Job drawing, mm, ordinate dimensions from the low corner. One solid piece. A direction names the side the tool comes from. Give positions to 0.01 mm unless a question says otherwise; leave off trailing zeros. Write each loop counter-clockwise with the first axis right and the second up, starting at its lowest first coordinate (ties: lowest second). Pieces come first, ordered by that corner, then holes. Notation, with made-up numbers: (37, 44.5) - (53, 44.5) arc R19 ccw to (53, 50.5) - close; hole circle Ø4 at (-16, 35). An arc over 180 degrees is marked (long way). Put each result on its own line as item: value. Start each with the question number.
1. Wall check: line 1 (Y direction, x = 131, z = 4.5); line 2 (X direction, y = 82, z = 46); line 3 (Z direction, x = 114, y = 110). Give the ranges that are in metal, low to high.
2. Cut at A-A on x = 74.5. List the corners of the cut face in (y, z).
3. Tool access for the marked faces 4 and 5: list every direction of +Z, -Z, +X, -X, +Y, -Y with a clear straight run to the whole face (end or side of a thin tool).
4. Cut at B-B on y = 38. List the corners of the cut face in (x, z), and give its area (3 significant figures).
5. Cut at C-C on z = 54. List the corners of the cut face in (x, y), and give its area (3 significant figures).
6. Cut at D-D on z = 74.5. List the corners of the cut face in (x, y), and give its area (3 significant figures).
7. Drop flat-ended pins along their axis: pin 1 (3 mm diameter, centred on x = 83.5, z = 85.5, fed in from -Y); pin 2 (6 mm diameter, centred on x = 105, y = 30, fed in from +Z). Give the stop position or say it passes through.
8. Mould opens along Y. For the marked faces 1, 2 and 3 say: +Y half, -Y half, draft (parallel to the pull), parting line (faces both ways), or undercut.
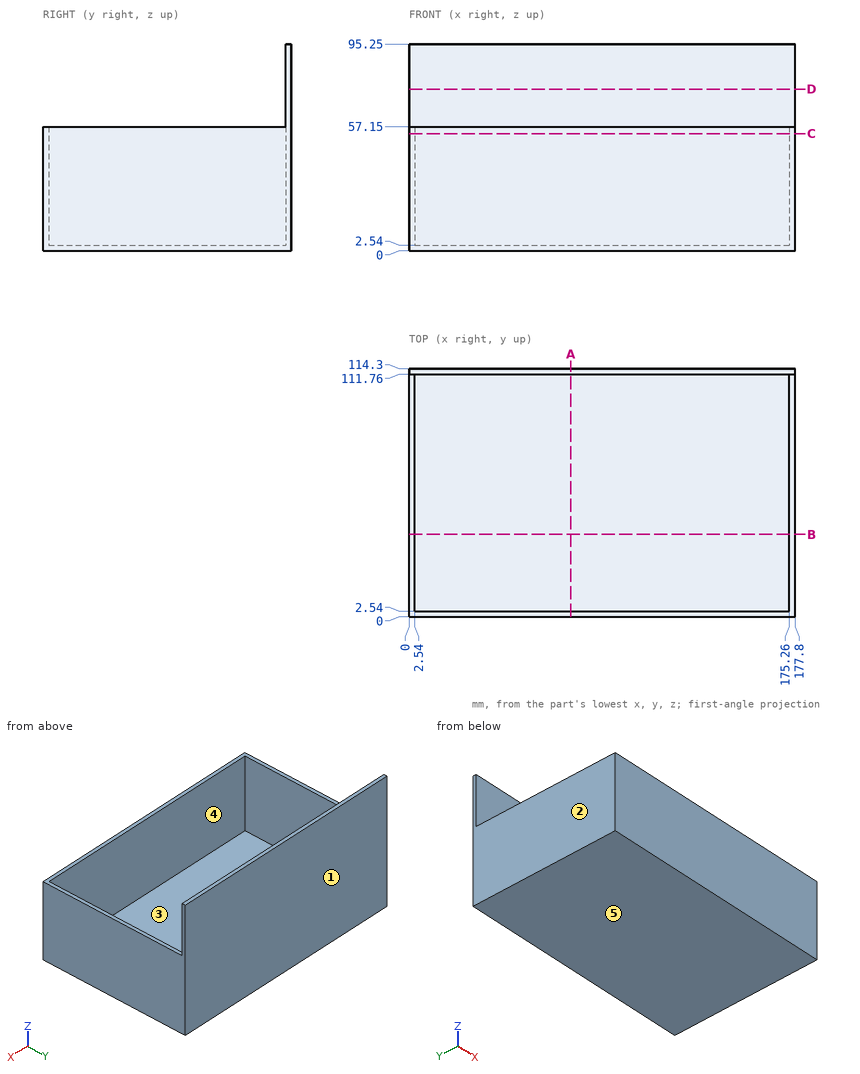
Report:
1. line 1: y = 0 to 2.54, 111.76 to 114.3
1. line 2: x = 0 to 2.54, 175.26 to 177.8
1. line 3: z = 0 to 2.54
2. outline: (0, 0) - (114.3, 0) - (114.3, 95.25) - (111.76, 95.25) - (111.76, 2.54) - (2.54, 2.54) - (2.54, 57.15) - (0, 57.15) - close
3. face 4: +Z
3. face 5: -Z, +X, -X, +Y, -Y
4. outline: (0, 0) - (177.8, 0) - (177.8, 57.15) - (175.26, 57.15) - (175.26, 2.54) - (2.54, 2.54) - (2.54, 57.15) - (0, 57.15) - close
4. area: 729 mm²
5. outline: (0, 0) - (177.8, 0) - (177.8, 114.3) - (0, 114.3) - close; hole (2.54, 2.54) - (175.26, 2.54) - (175.26, 111.76) - (2.54, 111.76) - close
5. area: 1,460 mm²
6. outline: (0, 111.76) - (177.8, 111.76) - (177.8, 114.3) - (0, 114.3) - close
6. area: 452 mm²
7. pin 1: stops at y = 111.76
7. pin 2: stops at z = 2.54
8. face 1: +Y half
8. face 2: draft
8. face 3: undercut
